```python
from build123d import *

# Parameters (mm, degrees)
BOSS_EXTRUDE1_DEPTH = 5
FILLET1_R           = 5


with BuildPart() as part:
    # Sketch1 → Boss-Extrude1 (new body)
    with BuildSketch(Plane.XY):
        Polygon((0, 60), (0, 55), (-5, 55), (-5, 50), (0, 50), (0, 46.5), (1, 46.5), (1, 47.6), (3.3, 47.6), (3.3, 46.5), (8, 46.5), (8, 43.5), (3.3, 43.5), (3.3, 42.4), (1, 42.4), (1, 43.5), (0, 43.5), (0, 40), (-5, 40), (-5, 35), (0, 35), (0, 25), (-5, 25), (-5, 20), (0, 20), (0, 16.5), (1, 16.5), (1, 17.6), (3.3, 17.6), (3.3, 16.5), (8, 16.5), (8, 13.5), (3.3, 13.5), (3.3, 12.4), (1, 12.4), (1, 13.5), (0, 13.5), (0, 10), (-5, 10), (-5, 5), (0, 5), (0, 0), (11, 0), (11, 60), align=None)
    extrude(amount=BOSS_EXTRUDE1_DEPTH)

    # Fillet1
    fillet1_edges = [part.edges().sort_by_distance(p)[0] for p in [
        (11, 60, 2.5),
        (11, 0, 2.5),
    ]]
    fillet(fillet1_edges, radius=FILLET1_R)


solid = part.part
```
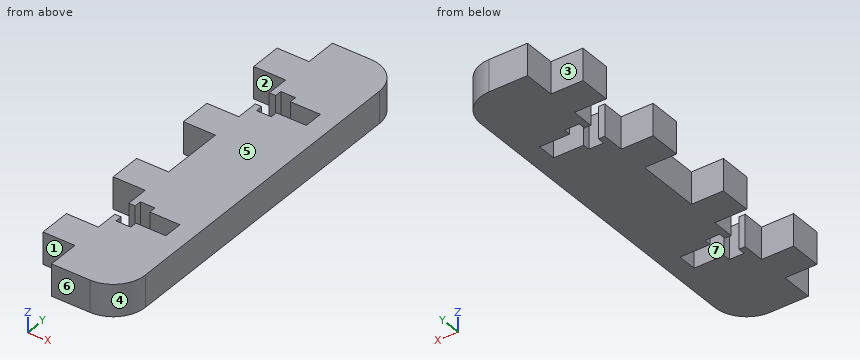
Geometry check sheet. Reference: the model listing, model coordinates, mm. Face numbers are marked on the shaded views. A direction names the side the tool comes from. Round coordinates to 2 decimals unless told otherwise and drop trailing zeros. Loops run counter-clockwise (first coordinate to the right, second up) from the corner with the lowest first, then second, coordinate; pieces in that order, holes last. Notation, with made-up numbers: (71, 82.25) - (108, 82.25) arc R12 ccw to (108, 98.25) - close; hole circle Ø3 at (-21.5, 14.5). An arc over 180 degrees is marked (long way). Use a Markdown table: item, result.
Q1. Material ranges on line 1 (Y direction, x = -3.75, z = 4.3); line 2 (Y direction, x = 2.5, z = 3.7); line 3 (Y direction, x = 3.75, z = 4.1), recorded low to high.
Solutions:
| item | result |
|---|---|
| line 1 | y = 5 to 10, 20 to 25, 35 to 40, 50 to 55 |
| line 2 | y = 0 to 12.4, 17.6 to 42.4, 47.6 to 60 |
| line 3 | y = 0 to 13.5, 16.5 to 43.5, 46.5 to 60 |
Q2. Cross-section at D-D on x = 2. Record the cut outline in (y, z).
Solutions:
| item | result |
|---|---|
| outline | (0, 0) - (12.4, 0) - (12.4, 5) - (0, 5) - close; (17.6, 0) - (42.4, 0) - (42.4, 5) - (17.6, 5) - close; (47.6, 0) - (60, 0) - (60, 5) - (47.6, 5) - close |
Q3. Cross-section at C-C on y = 28.5. Record the cut outline in (x, z).
Solutions:
| item | result |
|---|---|
| outline | (0, 0) - (11, 0) - (11, 5) - (0, 5) - close |
Q4. Go/stop test with flat-tipped pins: P1, Ø1, axis at y = 42.5, z = 2, coming from the -X side; P2, Ø1.5, axis at x = 8, z = 0.5, coming from the -Y side; P3, Ø2, axis at x = -3.5, z = 4, coming from the -Y side. Record where each tip stops, or that it passes through.
Solutions:
| item | result |
|---|---|
| P1 | stops at x = 0 |
| P2 | stops at y = 0.16 |
| P3 | stops at y = 5 |
Q5. Access from +Z, -Z, +X, -X, +Y, -Y to the whole of each face (thin tool, end or side, straight path). Record for the marked faces 1, 2, 3 and 4.
Solutions:
| item | result |
|---|---|
| face 1 | +Z, -Z, -X, -Y |
| face 2 | +Z, -Z, -X |
| face 3 | +Z, -Z, -X, +Y |
| face 4 | +Z, -Z, +X, -Y |
Q6. Cross-section at B-B on x = -1. Record the cut outline in (y, z).
Solutions:
| item | result |
|---|---|
| outline | (5, 0) - (10, 0) - (10, 5) - (5, 5) - close; (20, 0) - (25, 0) - (25, 5) - (20, 5) - close; (35, 0) - (40, 0) - (40, 5) - (35, 5) - close; (50, 0) - (55, 0) - (55, 5) - (50, 5) - close |
Q7. Draft check along Y on the marked faces 5, 6 and 7. Enter one of: released by +Y, released by -Y, zero draft, split by the parting line, or undercut.
Solutions:
| item | result |
|---|---|
| face 5 | zero draft |
| face 6 | released by -Y |
| face 7 | undercut |
Q8. Cross-section at A-A on x = 5. Record the cut outline in (y, z), plus the area to 3 significant figures.
Solutions:
| item | result |
|---|---|
| outline | (0, 0) - (13.5, 0) - (13.5, 5) - (0, 5) - close; (16.5, 0) - (43.5, 0) - (43.5, 5) - (16.5, 5) - close; (46.5, 0) - (60, 0) - (60, 5) - (46.5, 5) - close |
| area | 270 mm2 |
